Can you work these out from the drawing? Everything is in mm from the part's minimum corner. Give positions to 0.01 mm unless a question says otherwise; leave off trailing zeros. Order: outer loops, then holes, each group sorted by start corner. A loop starts at its lowest first (then second) coordinate and runs counter-clockwise, first axis right, second up. Notation, with made-up numbers: (-8, -33) -> (49, -33) arc R20 ccw to (49, -22) -> close; hole circle Ø5 at (-18.75, 89). An arc over 180 degrees is marked (long way). One line per item, written item: value.
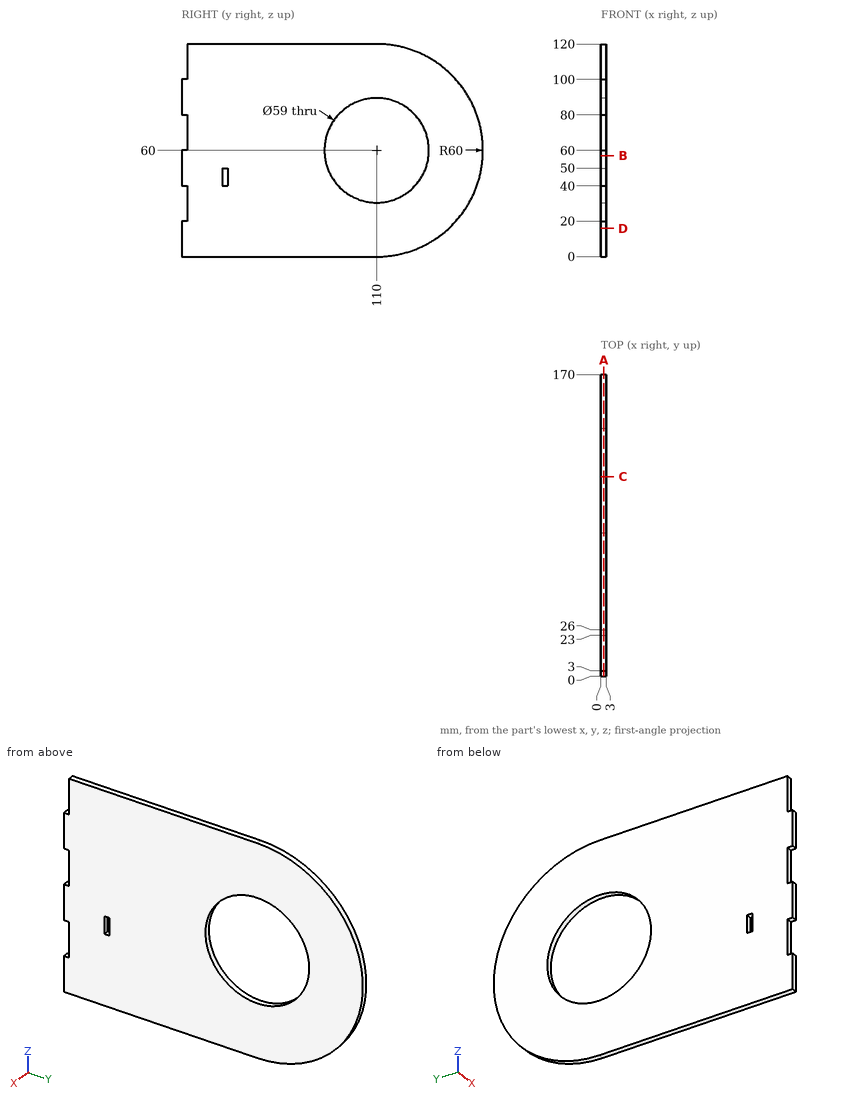
1) Suppose I cut it at A-A, the plane x = 1.6. Write out the boundary of the cut face in (y, z).
Answer below:
outline: (0, 0) -> (110, 0) arc R60 ccw to (110, 120) -> (3, 120) -> (3, 100) -> (0, 100) -> (0, 80) -> (3, 80) -> (3, 60) -> (0, 60) -> (0, 40) -> (3, 40) -> (3, 20) -> (0, 20) -> close; hole (23, 40) -> (26, 40) -> (26, 50) -> (23, 50) -> close; hole circle Ø59 at (110, 60)
2) For P1, Ø0.9, axis at x = 1, z = 46.5, coming from the +Y side; P2, Ø1.5, axis at x = 1.5, y = 1.5, coming from the +Z side; P3, Ø1.5, axis at x = 1.5, z = 107.5, coming from the -Y side, each with a flat end and sliding along its axis, tell me the tip position at first contact or that it passes through.
Answer below:
P1: stops at y = 168.56
P2: stops at z = 100
P3: stops at y = 3
3) If I drill on line 1 along Z through (x, y) = (2.7, 89); line 2 along Z through (x, y) = (0.5, 117); line 3 along Y through (x, z) = (1.95, 65), over which ranges is the centre line in solid material (lowest first)?
Answer below:
line 1: z = 0 to 39.28, 80.72 to 120
line 2: z = 0.41 to 31.34, 88.66 to 119.59
line 3: y = 3 to 80.93, 139.07 to 169.79
4) Suppose I cut it at C-C, the plane y = 112.5. Write out the boundary of the cut face in (x, z).
Answer below:
outline: (0, 0.05) -> (3, 0.05) -> (3, 30.61) -> (0, 30.61) -> close; (0, 89.39) -> (3, 89.39) -> (3, 119.95) -> (0, 119.95) -> close
5) Suppose I cut it at D-D, the plane z = 16. Write out the boundary of the cut face in (x, y).
Answer below:
outline: (0, 0) -> (3, 0) -> (3, 150.79) -> (0, 150.79) -> close
6) Suppose I cut it at B-B, the plane z = 57. Write out the boundary of the cut face in (x, y).
Answer below:
outline: (0, 0) -> (3, 0) -> (3, 80.65) -> (0, 80.65) -> close; (0, 139.35) -> (3, 139.35) -> (3, 169.92) -> (0, 169.92) -> close
